```python
from build123d import *

# Parameters (mm, degrees)
SKETCH1_R           = 13.575
SKETCH1_R_2         = 11.075
BOSS_EXTRUDE1_DEPTH = 7
FILLET1_R           = 0.5
FILLET2_R           = 0.5


with BuildPart() as part:
    # Sketch1 → Boss-Extrude1 (new body)
    with BuildSketch(Plane.XY):
        Circle(SKETCH1_R)
        Circle(SKETCH1_R_2, mode=Mode.SUBTRACT)
    extrude(amount=BOSS_EXTRUDE1_DEPTH)

    # Sketch2 → Cut-Revolve1 (revolve, cut)
    with BuildSketch(Plane(origin=(0, 0, 0), x_dir=(1, 0, 0), z_dir=(0, 1, 0)), mode=Mode.PRIVATE) as cut_revolve1_sk:
        Polygon((13.575, 0), (12.30110418, -3.5), (13.575, -7), align=None)
    revolve(cut_revolve1_sk.sketch.rotate(Axis((0, 0, 0), (0, 0, 1)), 180), axis=Axis((0, 0, 0), (0, 0, 1)), mode=Mode.SUBTRACT)

    # Fillet1
    fillet1_edges = [part.edges().sort_by_distance(p)[0] for p in [
        (13.575, 0, 7),
        (13.575, 0, 0),
    ]]
    fillet(fillet1_edges, radius=FILLET1_R)

    # Fillet2
    fillet2_edges = [part.edges().sort_by_distance(p)[0] for p in [
        (-11.075, 0, 0),
        (-11.075, 0, 7),
    ]]
    fillet(fillet2_edges, radius=FILLET2_R)


solid = part.part
```
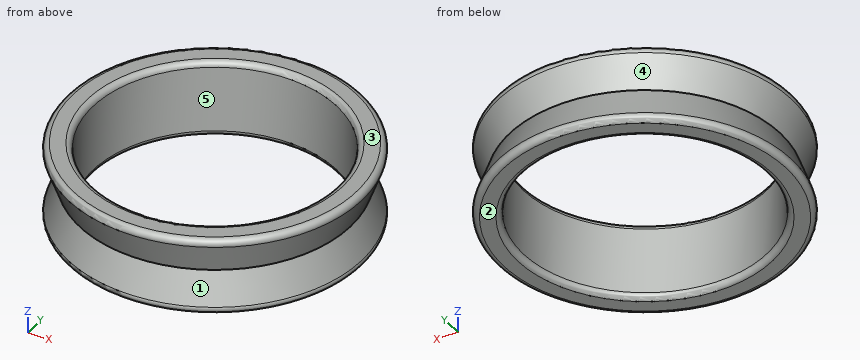
The model under review builds one solid part; all positions refer to its coordinate system, in mm. Face numbers are marked on the shaded views. A direction names the side the tool comes from. Give positions to 0.01 mm unless a question says otherwise; leave off trailing zeros. Write each loop counter-clockwise with the first axis right and the second up, starting at its lowest first coordinate (ties: lowest second). Pieces come first, ordered by that corner, then holes. Notation, with made-up numbers: M 8,-8 L 59,-8 A21 cw 59,25 Z; hole C 57.5,35 d5. An arc over 180 degrees is marked long. Write item = value, one per line. Start each with the question number.
Q1. We need section D-D (z = 1.75). State the section outline as (x, y) points (3 decimals), plus the area to 3 significant figures.
Q2. Clearance check with flat-ended pins moving along their axes: pin 1 (3 mm diameter, centred on y = -6, z = 5.5, fed in from +X); pin 2 (1.5 mm diameter, centred on y = 8, z = 3.5, fed in from +X); pin 3 (2 mm diameter, centred on y = 0.5, z = 2, fed in from -X). State where each tip first meets the part, or that it passes through.
Q3. Mouldability with a two-part tool opening along X and no side actions: class the marked faces 3, 4 and 5 as released by +X, released by -X, zero draft, split by the parting line, or undercut.
Q4. For line 1 (Y direction, x = -3.25, z = 4.5); line 2 (Y direction, x = 0, z = 3.95) (3 decimals); line 3 (Z direction, x = -8, y = 8.25), list the stretches that pass through material, from the lowest coordinate up.
Q5. We need section C-C (z = 4). State the section outline as (x, y) points (3 decimals).
Q6. We need section A-A (y = 0). State the section outline as (x, z) points (3 decimals), plus the area to 3 significant figures.
Q7. Machinability: for the marked faces 1 and 2, which of the approach directions +Z, -Z, +X, -X, +Y, -Y give a long, thin tool a straight path to every point of the face, cutting with its end or side? Answer none if there is none.
Result set:
q1.outline = C 0,0 d25.876; hole C 0,0 d22.15
q1.area = 141 mm2
q2.pin_1 = 12.46
q2.pin_2 = 10.03
q2.pin_3 = -13.2
q3.face_3 = zero draft
q3.face_4 = split by the parting line
q3.face_5 = undercut
q4.line_1 = -12.24 to -10.59, 10.59 to 12.24
q4.line_2 = -12.465 to -11.075, 11.075 to 12.465
q4.line_3 = 0.01 to 6.99
q5.outline = C 0,0 d24.966; hole C 0,0 d22.15
q6.outline = M -13.331,0.671 A0.5 ccw -12.861,0 L -11.575,0 A0.5 ccw -11.075,0.5 L -11.075,6.5 A0.5 ccw -11.575,7 L -12.861,7 A0.5 ccw -13.331,6.329 L -12.301,3.5 Z; M 11.075,0.5 A0.5 ccw 11.575,0 L 12.861,0 A0.5 ccw 13.331,0.671 L 12.301,3.5 L 13.331,6.329 A0.5 ccw 12.861,7 L 11.575,7 A0.5 ccw 11.075,6.5 Z
q6.area = 25.4 mm2
q7.face_1 = none
q7.face_2 = -Z, +X, -X, +Y, -Y
